from build123d import *

# Parameters (mm, degrees)
BOX002_W     = 37
BOX002_H     = 100
BOX002_DEPTH = 30
BOX003_W     = 86
BOX003_H     = 28
BOX003_DEPTH = 42
BOX004_W     = 86
BOX004_H     = 27.5
BOX004_DEPTH = 42
BOX001_W     = 37
BOX001_H     = 100
BOX001_DEPTH = 30
BOX_W        = 180
BOX_H        = 90
BOX_DEPTH    = 25
FILLET_R     = 5
FILLET001_R  = 5
FILLET002_R  = 7


with BuildPart() as cube002:
    # Box002 → Box002 (new body)
    with BuildSketch(Plane(origin=(133, -5, 13), x_dir=(1, 0, 0), z_dir=(0, 0, 1))):
        with Locations((18.5, 50)):
            Rectangle(BOX002_W, BOX002_H)
    extrude(amount=BOX002_DEPTH)


with BuildPart() as cube003:
    # Box003 → Box003 (new body)
    with BuildSketch(Plane(origin=(47, -1, -1), x_dir=(1, 0, 0), z_dir=(0, 0, 1))):
        with Locations((43, 14)):
            Rectangle(BOX003_W, BOX003_H)
    extrude(amount=BOX003_DEPTH)


with BuildPart() as cube004:
    # Box004 → Box004 (new body)
    with BuildSketch(Plane(origin=(47, 63.5, -1), x_dir=(1, 0, 0), z_dir=(0, 0, 1))):
        with Locations((43, 13.75)):
            Rectangle(BOX004_W, BOX004_H)
    extrude(amount=BOX004_DEPTH)


with BuildPart() as fusion:
    # Box001 → Box001 (new body)
    with BuildSketch(Plane(origin=(10, -5, 13), x_dir=(1, 0, 0), z_dir=(0, 0, 1))):
        with Locations((18.5, 50)):
            Rectangle(BOX001_W, BOX001_H)
    extrude(amount=BOX001_DEPTH)

    # Fusion: union Cube002, Cube003, Cube004
    add(cube002.part)
    add(cube003.part)
    add(cube004.part)


with BuildPart() as fillet002:
    # Box → Box (new body)
    with BuildSketch(Plane.XY):
        with Locations((90, 45)):
            Rectangle(BOX_W, BOX_H)
    extrude(amount=BOX_DEPTH)

    # Cut: cut Fusion
    add(fusion.part, mode=Mode.SUBTRACT)

    # Fillet
    fillet_edges = [fillet002.edges().sort_by_distance(p)[0] for p in [
        (10, 45, 13),
        (47, 45.25, 13),
        (133, 45.25, 13),
        (170, 45, 13),
    ]]
    fillet(fillet_edges, radius=FILLET_R)

    # Fillet001
    fillet001_edges = [fillet002.edges().sort_by_distance(p)[0] for p in [
        (90, 63.5, 0),
        (90, 27, 0),
    ]]
    fillet(fillet001_edges, radius=FILLET001_R)

    # Fillet002
    fillet002_edges = [fillet002.edges().sort_by_distance(p)[0] for p in [
        (90, 27, 25),
        (90, 63.5, 25),
    ]]
    fillet(fillet002_edges, radius=FILLET002_R)


solid = fillet002.part
The model under review builds one solid part; all positions refer to its coordinate system, in mm. A direction names the side the tool comes from. Round coordinates to 2 decimals unless told otherwise and drop trailing zeros. Write each loop counter-clockwise with the first axis right and the second up, starting at its lowest first coordinate (ties: lowest second). Pieces come first, ordered by that corner, then holes. Notation, with made-up numbers: (44.25, 24.25) - (54.25, 24.25) arc R16 ccw to (54.25, 35.25) - close; hole circle Ø3 at (70, -6). An arc over 180 degrees is marked (long way). One line per item, written item: value. Start each with the question number.
1. Consider section A-A on y = 84. Write out the cut boundary in (x, z).
2. Machinability: for faces 1 (the face through (133, 45, 21)), 2 (the face through (89, 29, 1)), 3 (the face through (89.4, 29.1, 23)), 4 (the face through (89.4, 62, 1.43)), 5 (the face through (161, 0, 10)), which of the approach directions +Z, -Z, +X, -X, +Y, -Y give a long, thin tool a straight path to every point of the face, cutting with its end or side? Answer none if there is none.
3. To check wall thickness, follow L1, parallel to X at y = 58.5, z = 18.25; L2, parallel to X at y = 65.5, z = 9.5; L3, parallel to X at y = 85, z = 20.25. State the ranges of each line that lie inside material, in increasing order. Write a range as from..to.
4. Consider section B-B on x = 83. Write out the cut boundary in (y, z), and give its area (3 significant figures).
5. Consider section D-D on y = 49.5. Write out the cut boundary in (x, z).
6. Clearance check with flat-ended pins moving along their axes: P1, Ø9.5, axis at x = 34.5, y = 42, coming from the +Z side; P2, Ø6.5, axis at x = 105, z = 11, coming from the -Y side; P3, Ø8, axis at x = 56.5, z = 9.5, coming from the +Y side. State where each tip first meets the part, or that it passes through.
7. Consider section C-C on z = 20.75. Write out the cut boundary in (x, y), and give its area (3 significant figures).
Checks:
1. outline: (0, 0) - (47, 0) - (47, 13) - (15, 13) arc R5 cw to (10, 18) - (10, 25) - (0, 25) - close; (133, 0) - (180, 0) - (180, 25) - (170, 25) - (170, 18) arc R5 cw to (165, 13) - (133, 13) - close
2. face 1: +Z, +Y, -Y
2. face 2: -Z, -Y
2. face 3: +Z, -Y
2. face 4: -Z, +Y
2. face 5: +Z, -Z, +X, -X, -Y
3. L1: x = 0..10, 47..133, 170..180
3. L2: x = 0..47, 133..180
3. L3: x = 0..10, 170..180
4. outline: (27, 5) arc R5 ccw to (32, 0) - (58.5, 0) arc R5 ccw to (63.5, 5) - (63.5, 18) arc R7 ccw to (56.5, 25) - (34, 25) arc R7 ccw to (27, 18) - close
4. area: 881 mm^2
5. outline: (0, 0) - (180, 0) - (180, 25) - (170, 25) - (170, 18) arc R5 cw to (165, 13) - (138, 13) arc R5 cw to (133, 18) - (133, 25) - (47, 25) - (47, 18) arc R5 cw to (42, 13) - (15, 13) arc R5 cw to (10, 18) - (10, 25) - (0, 25) - close
6. P1: stops at z = 13
6. P2: stops at y = 27
6. P3: stops at y = 63.5
7. outline: (0, 0) - (10, 0) - (10, 90) - (0, 90) - close; (47, 27.56) - (133, 27.56) - (133, 62.94) - (47, 62.94) - close; (170, 0) - (180, 0) - (180, 90) - (170, 90) - close
7. area: 4,840 mm^2
